Verification items for the finished model (mm, model axes). Face numbers are marked on the shaded views. A direction names the side the tool comes from. Round coordinates to 2 decimals unless told otherwise and drop trailing zeros. Write each loop counter-clockwise with the first axis right and the second up, starting at its lowest first coordinate (ties: lowest second). Pieces come first, ordered by that corner, then holes.
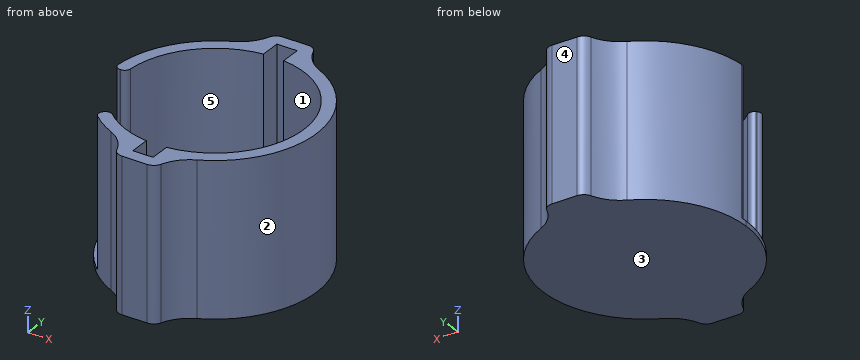
from build123d import *

# Parameters (mm, degrees)
F1_DEPTH    = 0.5999988
F2_DEPTH    = 19.05
F3_R        = 1.27
F4_R        = 5.08
F5_T1_DEPTH = 20.4776308939
F5_T3_DEPTH = 20.2938151504


# Not quite as in the source:
# - a fillet or chamfer that OpenCascade refuses, or shapes differently, is made with other operations: its cross-section is extruded or revolved along the edge and cut away or added


with BuildPart() as f1:
    # F0 (on Top) → F1 (new body)
    with BuildSketch(Plane.XY):
        with BuildLine():
            Line((-1.27, 13.5796900432), (-1.27, 11.0396900432))
            ThreePointArc((-1.27, 11.0396900432), (-8.2945925533, 7.3950923338), (-11.1125, 0))
            ThreePointArc((-11.1125, 0), (-10.266611305, -4.2525696422), (-7.8577241059, -7.8577241059))
            ThreePointArc((-7.8577241059, -7.8577241059), (-4.8332249736, -10.0063775966), (-1.27, -11.0396900432))
            Line((-1.27, -11.0396900432), (-1.27, -13.5796900432))
            Line((-1.27, -13.5796900432), (0, -13.5796900432))
            Line((0, -13.5796900432), (1.27, -13.5796900432))
            Line((1.27, -13.5796900432), (1.27, -11.0396900432))
            ThreePointArc((1.27, -11.0396900432), (11.1125, 0), (1.27, 11.0396900432))
            Line((1.27, 11.0396900432), (1.27, 13.5796900432))
            Line((1.27, 13.5796900432), (0, 13.5796900432))
            Line((0, 13.5796900432), (-1.27, 13.5796900432))
        make_face()
        with BuildLine():
            ThreePointArc((-7.8577241059, -7.8577241059), (-10.266611305, -4.2525696422), (-11.1125, 0))
            Line((-11.1125, 0), (-12.7, 0))
            ThreePointArc((-12.7, 0), (-11.7332700629, -4.860079591), (-8.9802561211, -8.9802561211))
            Line((-8.9802561211, -8.9802561211), (-7.8577241059, -7.8577241059))
        make_face()
    extrude(amount=F1_DEPTH)

    # F0 (on Top) → F2 (join)
    with BuildSketch(Plane.XY):
        with BuildLine():
            ThreePointArc((-11.1125, 0), (-8.2945925533, 7.3950923338), (-1.27, 11.0396900432))
            Line((-1.27, 11.0396900432), (-1.27, 13.5796900432))
            Line((-1.27, 13.5796900432), (0, 13.5796900432))
            Line((0, 13.5796900432), (1.27, 13.5796900432))
            Line((1.27, 13.5796900432), (1.27, 11.0396900432))
            ThreePointArc((1.27, 11.0396900432), (11.1125, 0), (1.27, -11.0396900432))
            Line((1.27, -11.0396900432), (1.27, -13.5796900432))
            Line((1.27, -13.5796900432), (0, -13.5796900432))
            Line((0, -13.5796900432), (-1.27, -13.5796900432))
            Line((-1.27, -13.5796900432), (-1.27, -11.0396900432))
            ThreePointArc((-1.27, -11.0396900432), (-4.8332249736, -10.0063775966), (-7.8577241059, -7.8577241059))
            Line((-7.8577241059, -7.8577241059), (-8.9802561211, -8.9802561211))
            ThreePointArc((-8.9802561211, -8.9802561211), (-6.1573611633, -11.1075156315), (-2.8575, -12.3743562964))
            Line((-2.8575, -12.3743562964), (-2.8575, -15.1671900432))
            Line((-2.8575, -15.1671900432), (0, -15.1671900432))
            Line((0, -15.1671900432), (2.8575, -15.1671900432))
            Line((2.8575, -15.1671900432), (2.8575, -12.3743562964))
            ThreePointArc((2.8575, -12.3743562964), (12.7, 0), (2.8575, 12.3743562964))
            Line((2.8575, 12.3743562964), (2.8575, 15.1671900432))
            Line((2.8575, 15.1671900432), (0, 15.1671900432))
            Line((0, 15.1671900432), (-2.8575, 15.1671900432))
            Line((-2.8575, 15.1671900432), (-2.8575, 12.3743562964))
            ThreePointArc((-2.8575, 12.3743562964), (-9.93932216, 7.9056862447), (-12.7, 0))
            Line((-12.7, 0), (-11.1125, 0))
        make_face()
    extrude(amount=F2_DEPTH)

    # F3
    f3_edges = [f1.edges().sort_by_distance(p)[0] for p in [
        (2.8575, -15.16719, 9.525),
        (-2.8575, -15.16719, 9.525),
        (-2.8575, 15.16719, 9.525),
        (2.8575, 15.16719, 9.525),
    ]]
    fillet(f3_edges, radius=F3_R)

    # F4
    f4_edges = [f1.edges().sort_by_distance(p)[0] for p in [
        (2.8575, 12.374356, 9.525),
        (-2.8575, 12.374356, 9.525),
        (-2.8575, -12.374356, 9.525),
        (2.8575, -12.374356, 9.525),
    ]]
    fillet(f4_edges, radius=F4_R)

    # F5: fillet of radius 0.762 on 4 edges, made by hand

    # F5_s2 → F5_t1 (cut)
    with BuildSketch(Plane.XY.offset(0.5999988)):
        with BuildLine():
            ThreePointArc((-12.6741021595, 0.8106382979), (-12.4694016476, 0.2406643993), (-11.91365603, 0))
            Line((-11.91365603, 0), (-12.7, 0))
            ThreePointArc((-12.7, 0), (-12.6935238887, 0.4055259388), (-12.6741021595, 0.8106382979))
        make_face()
        with BuildLine():
            ThreePointArc((-8.3887357449, -9.53515142), (-8.6470230336, -8.9873738911), (-8.4242269675, -8.4242269675))
            Line((-8.4242269675, -8.4242269675), (-8.9802561211, -8.9802561211))
            ThreePointArc((-8.9802561211, -8.9802561211), (-8.6889266776, -9.2624269601), (-8.3887357449, -9.53515142))
        make_face()
    extrude(amount=F5_T1_DEPTH, mode=Mode.SUBTRACT)

    # F5_s4 → F5_t3 (cut)
    with BuildSketch(Plane.XY.offset(0.5999988)):
        with BuildLine():
            ThreePointArc((-11.8500255801, 0), (-11.3287850299, 0.2061652325), (-11.0895961312, 0.7131016043))
            ThreePointArc((-11.0895961312, 0.7131016043), (-11.1067725568, 0.3567346651), (-11.1125, 0))
            Line((-11.1125, 0), (-11.8500255801, 0))
        make_face()
        with BuildLine():
            ThreePointArc((-8.379233445, -8.379233445), (-7.8648798833, -8.1564415512), (-7.3372896449, -8.345767605))
            ThreePointArc((-7.3372896449, -8.345767605), (-7.6014246912, -8.1059236928), (-7.8577241059, -7.8577241059))
            Line((-7.8577241059, -7.8577241059), (-8.379233445, -8.379233445))
        make_face()
    extrude(amount=F5_T3_DEPTH, mode=Mode.SUBTRACT)


solid = f1.part
Q1. Material ranges on line 1 along Z through (x, y) = (-3.5, -8); line 2 along X through (y, z) = (-8.5, 5.75); line 3 along Y through (x, z) = (-3.5, 8.5), recorded low to high.
Recorded:
line 1: z = 0 to 0.6
line 2: x = -8.49 to -7.16, 7.16 to 9.44
line 3: y = -13.02 to -10.55, 10.55 to 13.02
Q2. Sectioned sample at A-A (x = -0.5). Enter the section's corners in (y, z), plus the area to 3 significant figures.
Recorded:
outline: (-15.17, 0) - (15.17, 0) - (15.17, 19.05) - (13.58, 19.05) - (13.58, 0.6) - (-13.58, 0.6) - (-13.58, 19.05) - (-15.17, 19.05) - close
area: 76.8 mm2
Q3. Tool access check on the marked faces 4 and 5. Record the directions out of +Z, -Z, +X, -X, +Y, -Y that give a thin tool (end or side, any length) a straight path to the whole face; none if there is none.
Recorded:
face 4: +Z, -Z, +X, -X, +Y
face 5: +Z
Q4. Depth check by flat-ended pin: P1, Ø3, axis at x = -3, z = 10.5, coming from the +Y side; P2, Ø10, axis at y = -9.5, z = 15.5, coming from the -X side; P3, Ø2, axis at x = -3, y = 4.5, coming from the +Z side; P4, Ø1.3, axis at y = -12.5, z = 5.5, coming from the -X side. Enter the tip coordinate at first touch or a pass-through.
Recorded:
P1: stops at y = 15.17
P2: stops at x = -8.65
P3: stops at z = 0.6
P4: stops at x = -4.76
Q5. Release check for a two-part mould opening along X. For the marked faces 1, 2 and 3 record: released by +X, released by -X, zero draft, split by the parting line, or undercut.
Recorded:
face 1: undercut
face 2: released by +X
face 3: zero draft
Q6. Sectioned sample at B-B (y = 8). Enter the section's corners in (x, z).
Recorded:
outline: (-9.86, 0) - (9.86, 0) - (9.86, 19.05) - (7.71, 19.05) - (7.71, 0.6) - (-7.71, 0.6) - (-7.71, 19.05) - (-9.86, 19.05) - close
Q7. Sectioned sample at C-C (y = -3). Enter the section's corners in (x, z).
Recorded:
outline: (-12.34, 0) - (12.34, 0) - (12.34, 19.05) - (10.7, 19.05) - (10.7, 0.6) - (-12.34, 0.6) - close
